```python
from build123d import *

# Parameters (mm, degrees)
SKETCH1_R       = 2.286
MAIN_BODY_DEPTH = 1.5875


with BuildPart() as part:
    # Sketch1 → Main Body (new body)
    with BuildSketch(Plane(origin=(0, 0, 0), x_dir=(1, 0, 0), z_dir=(0, 1, 0))):
        Polygon((-25.4, 86.995), (-63.43142, 86.995), (-63.43142, 60.96), (-78.74, 60.96), (-78.74, 25.4), (-71.12, 25.4), (-71.12, -25.4), (-78.74, -25.4), (-78.74, -60.96), (-63.43142, -60.96), (-63.43142, -86.995), (-25.4, -86.995), (-25.4, -79.375), (25.4, -79.375), (25.4, -86.995), (63.43142, -86.995), (63.43142, -60.96), (78.74, -60.96), (78.74, -25.4), (71.12, -25.4), (71.12, 25.4), (78.74, 25.4), (78.74, 60.96), (63.43142, 60.96), (63.43142, 86.995), (25.4, 86.995), (25.4, 79.375), (-25.4, 79.375), align=None)
        with Locations((-57.15, 76.2)):
            Circle(SKETCH1_R, mode=Mode.SUBTRACT)
        with Locations((57.15, 76.2)):
            Circle(SKETCH1_R, mode=Mode.SUBTRACT)
        with Locations((57.15, -76.2)):
            Circle(SKETCH1_R, mode=Mode.SUBTRACT)
        with Locations((-57.15, -76.2)):
            Circle(SKETCH1_R, mode=Mode.SUBTRACT)
    extrude(amount=MAIN_BODY_DEPTH)


solid = part.part
```
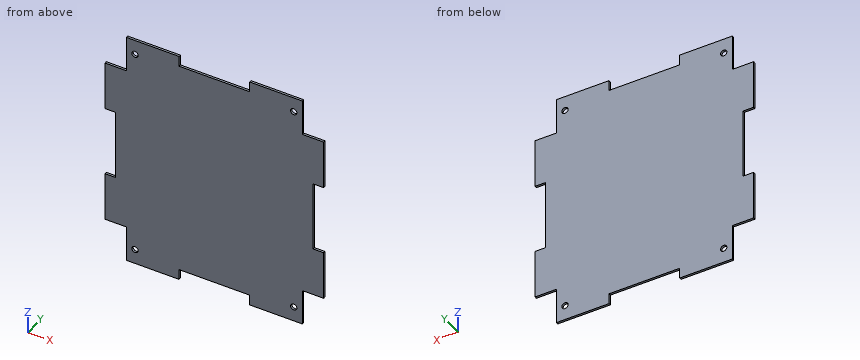
For this review, take the finished solid that the model builds, in its own axes (mm). Coordinates: 2 decimals unless noted, no trailing zeros. Write each loop counter-clockwise with the first axis right and the second up, starting at its lowest first coordinate (ties: lowest second). Pieces come first, ordered by that corner, then holes. Notation, with made-up numbers: (-14.5, -1.75) - (11.5, -1.75) arc R26 ccw to (11.5, 29.25) - close; hole circle Ø3 at (39.25, -1.5). An arc over 180 degrees is marked (long way). Answer in a Markdown table with one row per item. Add a question column.
Q1. For probe 1 along Z at (x, y) = (-57.15, 0.45) (3 decimals); probe 2 along X at (y, z) = (0.7, 76.2); probe 3 along X at (y, z) = (1.3, 78), list the stretches that pass through material, from the lowest coordinate up.
Q2. We need section B-B, the plane y = 1.1. Count the separate pieces of the cut face and the enclosed holes in it, and give its area (3 significant figures).
Q3. We need section C-C, the plane z = 76.2. State the section outline as (x, y) points, and give its area (3 significant figures).
Q4. We need section D-D, the plane z = -7.5. State the section outline as (x, y) points.
Q5. We need section A-A, the plane x = -57.15. State the section outline as (y, z) points (1 decimal).
Q6. For P1, Ø0.8, axis at x = -74.5, y = 0.5, coming from the +Z side; P2, Ø0.8, axis at y = 1, z = 70, coming from the +X side; P3, Ø0.5, axis at y = 1, z = 7, coming from the -X side; P4, Ø3.5, axis at x = -57.15, z = -76.2, coming from the -Y side, all flat-tipped, find the tip position at first contact; note any pin that passes through.
Answer list:
| question | item | result |
|---|---|---|
| 1 | probe 1 | z = -86.995 to -78.486, -73.914 to 73.914, 78.486 to 86.995 |
| 1 | probe 2 | x = -63.43 to -59.44, -54.86 to 54.86, 59.44 to 63.43 |
| 1 | probe 3 | x = -63.43 to -58.56, -55.74 to 55.74, 58.56 to 63.43 |
| 2 | separate pieces | 1 |
| 2 | enclosed holes | 4 |
| 2 | area | 24,200 mm2 |
| 3 | outline | (-63.43, 0) - (-59.44, 0) - (-59.44, 1.59) - (-63.43, 1.59) - close; (-54.86, 0) - (54.86, 0) - (54.86, 1.59) - (-54.86, 1.59) - close; (59.44, 0) - (63.43, 0) - (63.43, 1.59) - (59.44, 1.59) - close |
| 3 | area | 187 mm2 |
| 4 | outline | (-71.12, 0) - (71.12, 0) - (71.12, 1.59) - (-71.12, 1.59) - close |
| 5 | outline | (0, -87) - (1.6, -87) - (1.6, -78.5) - (0, -78.5) - close; (0, -73.9) - (1.6, -73.9) - (1.6, 73.9) - (0, 73.9) - close; (0, 78.5) - (1.6, 78.5) - (1.6, 87) - (0, 87) - close |
| 6 | P1 | stops at z = 60.96 |
| 6 | P2 | stops at x = 63.43 |
| 6 | P3 | stops at x = -71.12 |
| 6 | P4 | passes through |
